The figure shows three views and two pictorial views of one solid part (mm, origin at its lowest corner). Answer the questions. A direction names the side the tool comes from. Coordinates: 2 decimals unless noted, no trailing zeros. Loops run counter-clockwise (first coordinate to the right, second up) from the corner with the lowest first, then second, coordinate; pieces in that order, holes last. Notation, with made-up numbers: M 63,9.25 L 100,9.25 A29 cw 100,32.25 Z; hole C 16,-15.5 d1. An arc over 180 degrees is marked long. Return JSON: item names as keys, results as strings. Group by question number.
1. Which of the six approach directions +Z, -Z, +X, -X, +Y, -Y give full straight-line access (tool end or side, diameter ignored) to the marked faces 1 and 2?
2. Section D-D (z = 4.75) is taken. Write down the section's boundary in (x, y), then the cut area to 3 significant figures.
3. Section A-A (y = 1) is taken. Write down the section's boundary in (x, z).
4. Section B-B (x = 22.25) is taken. Write down the section's boundary in (y, z), then the cut area to 3 significant figures.
5. Section C-C (y = 6.25) is taken. Write down the section's boundary in (x, z).
6. The mould has two halves that part along Z. Classify the marked faces 3, 4 and 5: pulls with the +Z half, pulls with the -Z half, needs draft (parallel to the pull), parting line crosses it, or undercut.
7. Given P1, Ø0.8, axis at x = 28.5, y = 3, coming from the +Z side (3 decimals); P2, Ø3, axis at x = 20, z = 8.5, coming from the -Y side; P3, Ø1.1, axis at y = 0.5, z = 13.5, coming from the -X side, each flat-ended and moving along its own axis, determine where each tip first touches the part or whether it passes through.
8. Straight lines are drawn through the part: L1, parallel to X at y = 4.5, z = 6.75; L2, parallel to Z at x = 22, y = 1.25; L3, parallel to Z at x = 10.5, y = 5.5. For each, find the intervals that lie inside material, in ascending order. Write a range as from..to.
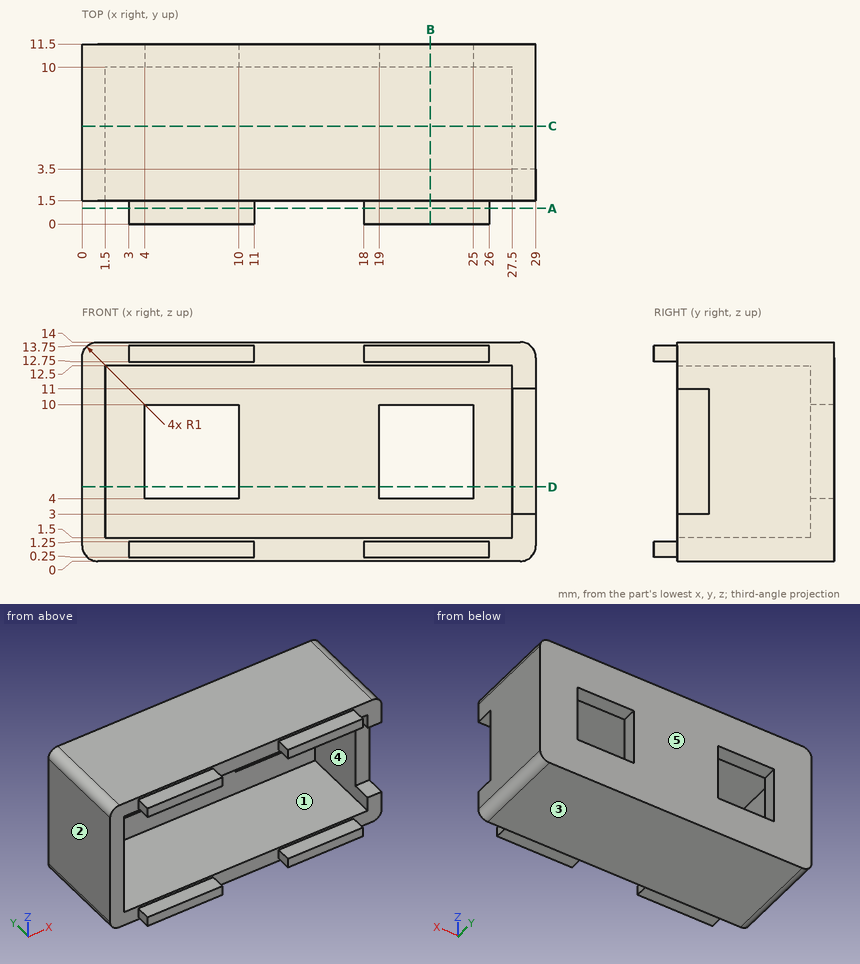
Worked out:
{
 "1": {"face 1": "-Y", "face 2": "+Z, -Z, -X, +Y, -Y"},
 "2": {"outline": "M 0,1.5 L 1.5,1.5 L 1.5,10 L 4,10 L 4,11.5 L 0,11.5 Z; M 10,10 L 19,10 L 19,11.5 L 10,11.5 Z; M 25,10 L 27.5,10 L 27.5,3.5 L 29,3.5 L 29,11.5 L 25,11.5 Z", "area": "48.0 mm^2"},
 "3": {"outline": "M 3,0.25 L 11,0.25 L 11,1.25 L 3,1.25 Z; M 3,12.75 L 11,12.75 L 11,13.75 L 3,13.75 Z; M 18,0.25 L 26,0.25 L 26,1.25 L 18,1.25 Z; M 18,12.75 L 26,12.75 L 26,13.75 L 18,13.75 Z"},
 "4": {"outline": "M 0,0.25 L 1.5,0.25 L 1.5,0 L 11.5,0 L 11.5,4 L 10,4 L 10,1.5 L 1.5,1.5 L 1.5,1.25 L 0,1.25 Z; M 0,12.75 L 1.5,12.75 L 1.5,12.5 L 10,12.5 L 10,10 L 11.5,10 L 11.5,14 L 1.5,14 L 1.5,13.75 L 0,13.75 Z", "area": "40.5 mm^2"},
 "5": {"outline": "M 0,1 A1 ccw 1,0 L 28,0 A1 ccw 29,1 L 29,13 A1 ccw 28,14 L 1,14 A1 ccw 0,13 Z; hole M 1.5,1.5 L 27.5,1.5 L 27.5,12.5 L 1.5,12.5 Z"},
 "6": {"face 3": "pulls with the -Z half", "face 4": "undercut", "face 5": "needs draft"},
 "7": {"P1": "z = 13.995", "P2": "y = 10", "P3": "x = 3"},
 "8": {"L1": "0..1.5, 27.5..29", "L2": "0.25..1.25, 12.75..13.75", "L3": "0..1.5, 12.5..14"}
}
